Autodesk Inventor part; units mm, degrees
ref_plane "YZ Plane" through (0, 0, 0) normal (1, 0, 0) x (0, 1, 0)
ref_plane "XZ Plane" through (0, 0, 0) normal (0, 1, 0) x (-1, 0, 0)
ref_plane "XY Plane" through (0, 0, 0) normal (0, 0, 1) x (1, 0, 0)
sketch "Sketch1" plane through (0, 0, 0) normal (0, 1, 0) x (-1, 0, 0)
  line L0 (0, 0) -> (-10.16, 0)
  line L1 (-10.16, 0) -> (-10.16, -76.2)
  line L2 (-10.16, -76.2) -> (0, -76.2)
  line L3 (0, -76.2) -> (0, 0)
  line L4 (-5.08, -76.2) -> (-5.08, 0) construction
  circle A0 centre (-5.08, -71.12) radius 1.5
  circle A1 centre (-5.08, -5.08) radius 1.5
  dimension "d0" = 10.16
  dimension "d1" = 76.2
  dimension "d2" = 3
  dimension "d3" = 3
  dimension "d4" = 5.08
  dimension "d5" = 5.08
extrude "Extrusion1" add sketch "Sketch1" along normal blind 5
fillet "Fillet1" radius 5.08 4 edges at (10.16, 2.5, 0) (0, 2.5, 0) (10.16, 2.5, -76.2) (0, 2.5, -76.2)
chamfer "Chamfer1" distance 0.635 angle 45 12 edges at (10.16, 5, -38.1) (8.6721, 5, -74.7121) (8.6721, 5, -1.4879) (0, 5, -38.1) (1.4879, 5, -1.4879) (1.4879, 5, -74.7121) (10.16, 0, -38.1) (8.6721, 0, -74.7121) (8.6721, 0, -1.4879) (1.4879, 0, -1.4879) (0, 0, -38.1) (1.4879, 0, -74.7121)
equation "\"d4\" = 0.5 * d0"
equation "\"d5\" = d4"
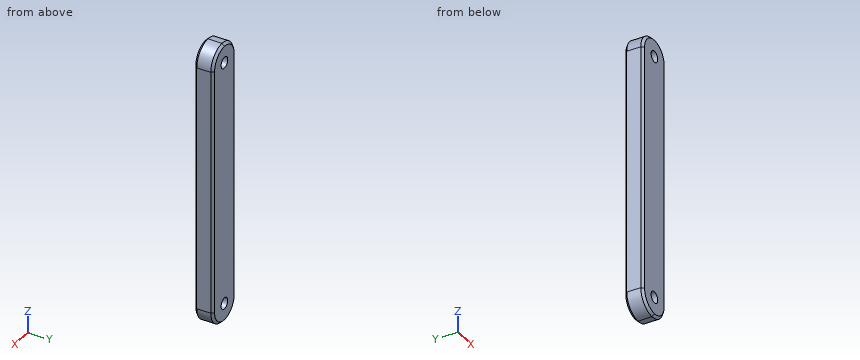
Can you work these out from the model? Positions are in its coordinate system, mm. Give positions to 0.01 mm unless a question says otherwise; leave off trailing zeros. Write each loop counter-clockwise with the first axis right and the second up, starting at its lowest first coordinate (ties: lowest second). Pieces come first, ordered by that corner, then holes. Notation, with made-up numbers: (28.5, 80) -> (69.5, 80) arc R20 ccw to (69.5, 87) -> close; hole circle Ø9 at (67, -38). An arc over 180 degrees is marked (long way). Write item = value, one per line.
(1) I need wall thicknesses on probe 1 along Z at (x, y) = (5.08, 3.45); probe 2 along Z at (x, y) = (4, 3.9); probe 3 along X at (y, z) = (2.5, -71.12). Which ranges of each line are inside material? Lowest first, please. Write a range as from..to.
Worked out:
probe_1 = -76.2..-72.62, -69.62..-6.58, -3.58..0
probe_2 = -76.08..-72.16, -70.08..-6.12, -4.04..-0.12
probe_3 = 0..3.58, 6.58..10.16
(2) Suppose I cut it at A-A on y = 1.35. Count the separate pieces of the cut face and the enclosed holes in it, then the cut area to 3 significant figures.
Worked out:
separate_pieces = 1
enclosed_holes = 2
area = 738 mm^2
(3) Suppose I cut it at B-B on z = -17. Write out the boundary of the cut face in (x, y) (3 decimals).
Worked out:
outline = (0, 0.635) -> (0.635, 0) -> (9.525, 0) -> (10.16, 0.635) -> (10.16, 4.365) -> (9.525, 5) -> (0.635, 5) -> (0, 4.365) -> close
(4) I'm going to push flat-ended pins straight in: P1, Ø1.5, axis at x = 4, y = 4.5, coming from the +Z side; P2, Ø3, axis at x = 1.5, y = 2.5, coming from the -Z side. Where does each tip first touch, or does it pass through?
Worked out:
P1 = -0.01
P2 = -75.75
